Check sheet for the modelled part. Datum: model origin and axes. Units: mm. A direction names the side the tool comes from. Round coordinates to 2 decimals unless told otherwise and drop trailing zeros. Order: outer loops, then holes, each group sorted by start corner. A loop starts at its lowest first (then second) coordinate and runs counter-clockwise, first axis right, second up. Notation, with made-up numbers: (-27, 10.25) -> (-3, 10.25) arc R34 ccw to (-3, 44.25) -> close; hole circle Ø10 at (40, 73.25). An arc over 180 degrees is marked (long way). Answer in a Markdown table with one row per item. Add a question column.
1. Access from +Z, -Z, +X, -X, +Y, -Y to the whole of each face (thin tool, end or side, straight path). Record for faces 4 (the flat face through (7, 5, -7.5)), 5 (the cylindrical face through (31.21, 2.96, -17.94)).
2. Draft check along X on faces 1 (the cylindrical face through (-21.28, 2.96, 21.15)), 2 (the flat face through (-19, 6, 0)), 3 (the cylindrical face through (-31.21, 2.96, 17.94)). Enter one of: +X half, -X half, draft (parallel to the pull), parting line (faces both ways), or undercut.
3. Material ranges on L1, parallel to X at y = 1.05, z = -30; L2, parallel to Z at x = 16, y = 4.3; L3, parallel to Z at x = 30.5, y = 2.4, recorded low to high. Write a range as from..to.
4. Sectioned sample at A-A, the plane y = 2.3. Record the boundary of the cut face in (x, z).
5. Depth check by flat-ended pin: P1, Ø2, axis at y = 4.5, z = 10, coming from the -X side; P2, Ø1.9, axis at y = 5, z = 4, coming from the +X side; P3, Ø1, axis at y = 4.5, z = -2.5, coming from the -X side. Enter the tip coordinate at first touch or a pass-through.
6. Sectioned sample at B-B, the plane x = 7. Record the boundary of the cut face in (y, z), then the cut area to 3 significant figures.
```python
from build123d import *

# Parameters (mm, degrees)
BOSS_EXTRUDE1_DEPTH = 4
BOSS_EXTRUDE3_DEPTH = 2
CUT_EXTRUDE1_DEPTH  = 2
SKETCH2_R           = 26
SKETCH2_R_2         = 24
BOSS_EXTRUDE4_DEPTH = 2
SKETCH5_W           = 30
SKETCH5_H           = 15
SKETCH5_R           = 4
SKETCH5_R_2         = 2
BOSS_EXTRUDE5_DEPTH = 2
BOSS_EXTRUDE6_DEPTH = 2
CUT_EXTRUDE2_DEPTH  = 2
SKETCH8_R           = 2
CUT_EXTRUDE3_DEPTH  = 6
FILLET1_R           = 2


with BuildPart() as part:
    # Sketch1 → Boss-Extrude1 (new body)
    with BuildSketch(Plane(origin=(0, 0, 0), x_dir=(1, 0, 0), z_dir=(0, 1, 0))):
        with BuildLine():
            ThreePointArc((31.766819559, 13.412064474), (28.977774789, 7.764571353), (34.216904973, 4.268221228))
            ThreePointArc((34.216904973, 4.268221228), (36, 0), (34.216904973, -4.268221228))
            ThreePointArc((34.216904973, -4.268221228), (28.977774789, -7.764571353), (31.766819559, -13.412064474))
            ThreePointArc((31.766819559, -13.412064474), (31.176914536, -18), (27.498598332, -20.804840499))
            ThreePointArc((27.498598332, -20.804840499), (21.213203436, -21.213203436), (20.804840499, -27.498598332))
            ThreePointArc((20.804840499, -27.498598332), (18, -31.176914536), (13.412064474, -31.766819559))
            ThreePointArc((13.412064474, -31.766819559), (7.764571353, -28.977774789), (4.268221228, -34.216904973))
            ThreePointArc((4.268221228, -34.216904973), (0, -36), (-4.268221228, -34.216904973))
            ThreePointArc((-4.268221228, -34.216904973), (-7.764571353, -28.977774789), (-13.412064474, -31.766819559))
            ThreePointArc((-13.412064474, -31.766819559), (-18, -31.176914536), (-20.804840499, -27.498598332))
            ThreePointArc((-20.804840499, -27.498598332), (-21.213203436, -21.213203436), (-27.498598332, -20.804840499))
            ThreePointArc((-27.498598332, -20.804840499), (-31.176914536, -18), (-31.766819559, -13.412064474))
            ThreePointArc((-31.766819559, -13.412064474), (-28.977774789, -7.764571353), (-34.216904973, -4.268221228))
            ThreePointArc((-34.216904973, -4.268221228), (-36, 0), (-34.216904973, 4.268221228))
            ThreePointArc((-34.216904973, 4.268221228), (-28.977774789, 7.764571353), (-31.766819559, 13.412064474))
            ThreePointArc((-31.766819559, 13.412064474), (-31.176914536, 18), (-27.498598332, 20.804840499))
            ThreePointArc((-27.498598332, 20.804840499), (-21.213203436, 21.213203436), (-20.804840499, 27.498598332))
            ThreePointArc((-20.804840499, 27.498598332), (-18, 31.176914536), (-13.412064474, 31.766819559))
            ThreePointArc((-13.412064474, 31.766819559), (-7.764571353, 28.977774789), (-4.268221228, 34.216904973))
            ThreePointArc((-4.268221228, 34.216904973), (0, 36), (4.268221228, 34.216904973))
            ThreePointArc((4.268221228, 34.216904973), (7.764571353, 28.977774789), (13.412064474, 31.766819559))
            ThreePointArc((13.412064474, 31.766819559), (18, 31.176914536), (20.804840499, 27.498598332))
            ThreePointArc((20.804840499, 27.498598332), (21.213203436, 21.213203436), (27.498598332, 20.804840499))
            ThreePointArc((27.498598332, 20.804840499), (31.176914536, 18), (31.766819559, 13.412064474))
        make_face()
    extrude(amount=BOSS_EXTRUDE1_DEPTH)

    # Sketch4 → Boss-Extrude3 (add)
    with BuildSketch(Plane(origin=(0, 4, 0), x_dir=(1, 0, 0), z_dir=(0, 1, 0))):
        with BuildLine():
            ThreePointArc((-13.412064474, 31.766819559), (-18, 31.176914536), (-20.804840499, 27.498598332))
            ThreePointArc((-20.804840499, 27.498598332), (-21.213203436, 21.213203436), (-27.498598332, 20.804840499))
            ThreePointArc((-27.498598332, 20.804840499), (-31.176914536, 18), (-31.766819559, 13.412064474))
            ThreePointArc((-31.766819559, 13.412064474), (-28.977774789, 7.764571353), (-34.216904973, 4.268221228))
            ThreePointArc((-34.216904973, 4.268221228), (-36, 0), (-34.216904973, -4.268221228))
            ThreePointArc((-34.216904973, -4.268221228), (-28.977774789, -7.764571353), (-31.766819559, -13.412064474))
            ThreePointArc((-31.766819559, -13.412064474), (-31.176914536, -18), (-27.498598332, -20.804840499))
            ThreePointArc((-27.498598332, -20.804840499), (-21.213203436, -21.213203436), (-20.804840499, -27.498598332))
            ThreePointArc((-20.804840499, -27.498598332), (-18, -31.176914536), (-13.412064474, -31.766819559))
            ThreePointArc((-13.412064474, -31.766819559), (-7.764571353, -28.977774789), (-4.268221228, -34.216904973))
            ThreePointArc((-4.268221228, -34.216904973), (0, -36), (4.268221228, -34.216904973))
            ThreePointArc((4.268221228, -34.216904973), (7.764571353, -28.977774789), (13.412064474, -31.766819559))
            ThreePointArc((13.412064474, -31.766819559), (18, -31.176914536), (20.804840499, -27.498598332))
            ThreePointArc((20.804840499, -27.498598332), (21.213203436, -21.213203436), (27.498598332, -20.804840499))
            ThreePointArc((27.498598332, -20.804840499), (31.176914536, -18), (31.766819559, -13.412064474))
            ThreePointArc((31.766819559, -13.412064474), (28.977774789, -7.764571353), (34.216904973, -4.268221228))
            ThreePointArc((34.216904973, -4.268221228), (36, 0), (34.216904973, 4.268221228))
            ThreePointArc((34.216904973, 4.268221228), (28.977774789, 7.764571353), (31.766819559, 13.412064474))
            ThreePointArc((31.766819559, 13.412064474), (31.176914536, 18), (27.498598332, 20.804840499))
            ThreePointArc((27.498598332, 20.804840499), (21.213203436, 21.213203436), (20.804840499, 27.498598332))
            ThreePointArc((20.804840499, 27.498598332), (18, 31.176914536), (13.412064474, 31.766819559))
            ThreePointArc((13.412064474, 31.766819559), (7.764571353, 28.977774789), (4.268221228, 34.216904973))
            ThreePointArc((4.268221228, 34.216904973), (0, 36), (-4.268221228, 34.216904973))
            ThreePointArc((-4.268221228, 34.216904973), (-7.764571353, 28.977774789), (-13.412064474, 31.766819559))
        make_face()
    extrude(amount=BOSS_EXTRUDE3_DEPTH)

    # Sketch3 → Cut-Extrude1 (cut)
    with BuildSketch(Plane(origin=(0, 4, 0), x_dir=(1, 0, 0), z_dir=(0, 1, 0))):
        with BuildLine():
            ThreePointArc((-14.726691345, 29.971413987), (-17, 29.444863729), (-18.592660228, 27.739395812))
            ThreePointArc((-18.592660228, 27.739395812), (-19.798989873, 19.798989873), (-27.739395812, 18.592660228))
            ThreePointArc((-27.739395812, 18.592660228), (-29.444863729, 17), (-29.971413987, 14.726691345))
            ThreePointArc((-29.971413987, 14.726691345), (-27.045923136, 7.246933263), (-33.319351573, 2.232018175))
            ThreePointArc((-33.319351573, 2.232018175), (-34, 0), (-33.319351573, -2.232018175))
            ThreePointArc((-33.319351573, -2.232018175), (-27.045923136, -7.246933263), (-29.971413987, -14.726691345))
            ThreePointArc((-29.971413987, -14.726691345), (-29.444863729, -17), (-27.739395812, -18.592660228))
            ThreePointArc((-27.739395812, -18.592660228), (-19.798989873, -19.798989873), (-18.592660228, -27.739395812))
            ThreePointArc((-18.592660228, -27.739395812), (-17, -29.444863729), (-14.726691345, -29.971413987))
            ThreePointArc((-14.726691345, -29.971413987), (-7.246933263, -27.045923136), (-2.232018175, -33.319351573))
            ThreePointArc((-2.232018175, -33.319351573), (0, -34), (2.232018175, -33.319351573))
            ThreePointArc((2.232018175, -33.319351573), (7.246933263, -27.045923136), (14.726691345, -29.971413987))
            ThreePointArc((14.726691345, -29.971413987), (17, -29.444863729), (18.592660228, -27.739395812))
            ThreePointArc((18.592660228, -27.739395812), (19.798989873, -19.798989873), (27.739395812, -18.592660228))
            ThreePointArc((27.739395812, -18.592660228), (29.444863729, -17), (29.971413987, -14.726691345))
            ThreePointArc((29.971413987, -14.726691345), (27.045923136, -7.246933263), (33.319351573, -2.232018175))
            ThreePointArc((33.319351573, -2.232018175), (34, 0), (33.319351573, 2.232018175))
            ThreePointArc((33.319351573, 2.232018175), (27.045923136, 7.246933263), (29.971413987, 14.726691345))
            ThreePointArc((29.971413987, 14.726691345), (29.444863729, 17), (27.739395812, 18.592660228))
            ThreePointArc((27.739395812, 18.592660228), (19.798989873, 19.798989873), (18.592660228, 27.739395812))
            ThreePointArc((18.592660228, 27.739395812), (17, 29.444863729), (14.726691345, 29.971413987))
            ThreePointArc((14.726691345, 29.971413987), (7.246933263, 27.045923136), (2.232018175, 33.319351573))
            ThreePointArc((2.232018175, 33.319351573), (0, 34), (-2.232018175, 33.319351573))
            ThreePointArc((-2.232018175, 33.319351573), (-7.246933263, 27.045923136), (-14.726691345, 29.971413987))
        make_face()
    extrude(amount=CUT_EXTRUDE1_DEPTH, mode=Mode.SUBTRACT)

    # Sketch2 → Boss-Extrude4 (add)
    with BuildSketch(Plane(origin=(0, 4, 0), x_dir=(1, 0, 0), z_dir=(0, 1, 0))):
        with Locations(Location((0, 0, 0), (0, 0, 270))):
            Circle(SKETCH2_R)
        with Locations(Location((0, 0, 0), (0, 0, 270))):
            Circle(SKETCH2_R_2, mode=Mode.SUBTRACT)
    extrude(amount=BOSS_EXTRUDE4_DEPTH)

    # Sketch5 → Boss-Extrude5 (add)
    # profile 1 of 5: a face of its own
    with BuildSketch(Plane(origin=(0, 4, 0), x_dir=(1, 0, 0), z_dir=(0, 1, 0))):
        with BuildLine():
            Line((-17, 5), (-17, -5))
            ThreePointArc((-17, -5), (-22, 0), (-17, 5))
        make_face()
    # profile 2 of 5: a face of its own
    with BuildSketch(Plane(origin=(0, 4, 0), x_dir=(1, 0, 0), z_dir=(0, 1, 0))):
        Rectangle(SKETCH5_W, SKETCH5_H)
        with Locations(Location((-7, 0, 0), (0, 0, 270))):
            Circle(SKETCH5_R, mode=Mode.SUBTRACT)
        with Locations(Location((7, 0, 0), (0, 0, 270))):
            Circle(SKETCH5_R, mode=Mode.SUBTRACT)
    # profile 3 of 5: a face of its own
    with BuildSketch(Plane(origin=(0, 4, 0), x_dir=(1, 0, 0), z_dir=(0, 1, 0))):
        with Locations(Location((-7, 0, 0), (0, 0, 270))):
            Circle(SKETCH5_R_2)
    # profile 4 of 5: a face of its own
    with BuildSketch(Plane(origin=(0, 4, 0), x_dir=(1, 0, 0), z_dir=(0, 1, 0))):
        with Locations(Location((7, 0, 0), (0, 0, 270))):
            Circle(SKETCH5_R_2)
    # profile 5 of 5: a face of its own
    with BuildSketch(Plane(origin=(0, 4, 0), x_dir=(1, 0, 0), z_dir=(0, 1, 0))):
        with BuildLine():
            ThreePointArc((17, 5), (22, 0), (17, -5))
            Line((17, -5), (17, 5))
        make_face()
    extrude(amount=BOSS_EXTRUDE5_DEPTH)

    # Sketch6 → Boss-Extrude6 (add)
    with BuildSketch(Plane(origin=(0, 4, 0), x_dir=(1, 0, 0), z_dir=(0, 1, 0))):
        with BuildLine():
            Line((0, 7.5), (1.907283427, 12.740218147))
            ThreePointArc((1.907283427, 12.740218147), (4.07818129, 15.957233587), (3.67332787, 12.097430538))
            Line((3.67332787, 12.097430538), (2, 7.5))
            Line((2, 7.5), (0, 7.5))
        make_face()
    extrude(amount=BOSS_EXTRUDE6_DEPTH)

    # Sketch7 → Cut-Extrude2 (cut)
    with BuildSketch(Plane(origin=(0, 6, 0), x_dir=(1, 0, 0), z_dir=(0, 1, 0))):
        with BuildLine():
            Line((2.126154469, -3.388136239), (2.510116854, -4))
            Line((2.510116854, -4), (2.973799982, -4.738902857))
            ThreePointArc((2.973799982, -4.738902857), (0.649911516, -5.55682478), (-1.8, -5.297233865))
            Line((-1.8, -5.297233865), (-1.8, -3.57211422))
            ThreePointArc((-1.8, -3.57211422), (0.1872329, -3.995615577), (2.126154469, -3.388136239))
        make_face()
    extrude(amount=-CUT_EXTRUDE2_DEPTH, mode=Mode.SUBTRACT)

    # Sketch8 → Cut-Extrude3 (cut)
    with BuildSketch(Plane(origin=(0, 4, 0), x_dir=(1, 0, 0), z_dir=(0, 1, 0))):
        with Locations(Location((0, 30, 0), (0, 0, 270))):
            Circle(SKETCH8_R)
    extrude(amount=-CUT_EXTRUDE3_DEPTH, mode=Mode.SUBTRACT)

    # Fillet1
    fillet1_edges = [part.edges().sort_by_distance(p)[0] for p in [
        (-15, 5, 7.5),
        (15, 5, 7.5),
        (15, 5, -7.5),
        (-15, 5, -7.5),
    ]]
    fillet(fillet1_edges, radius=FILLET1_R)


solid = part.part
```
Answer key:
| question | item | result |
|---|---|---|
| 1 | face 4 | +Y |
| 1 | face 5 | +X, +Y, -Y |
| 2 | face 1 | undercut |
| 2 | face 2 | draft |
| 2 | face 3 | -X half |
| 3 | L1 | x = -19.45..-12.15, -5.85..-2, 2..5.85, 12.15..19.45 |
| 3 | L2 | z = -31.9..-29.85, -20.49..-17.89, 17.89..20.49, 29.85..31.9 |
| 3 | L3 | z = -18.95..-12.64, -5.36..5.36, 12.64..18.95 |
| 4 | outline | (-34.22, -4.27) arc R4.77 cw to (-31.77, -13.41) arc R6 ccw to (-27.5, -20.8) arc R4.77 cw to (-20.8, -27.5) arc R6 ccw to (-13.41, -31.77) arc R4.77 cw to (-4.27, -34.22) arc R6 ccw to (4.27, -34.22) arc R4.77 cw to (13.41, -31.77) arc R6 ccw to (20.8, -27.5) arc R4.77 cw to (27.5, -20.8) arc R6 ccw to (31.77, -13.41) arc R4.77 cw to (34.22, -4.27) arc R6 ccw to (34.22, 4.27) arc R4.77 cw to (31.77, 13.41) arc R6 ccw to (27.5, 20.8) arc R4.77 cw to (20.8, 27.5) arc R6 ccw to (13.41, 31.77) arc R4.77 cw to (4.27, 34.22) arc R6 ccw to (-4.27, 34.22) arc R4.77 cw to (-13.41, 31.77) arc R6 ccw to (-20.8, 27.5) arc R4.77 cw to (-27.5, 20.8) arc R6 ccw to (-31.77, 13.41) arc R4.77 cw to (-34.22, 4.27) arc R6 ccw to start; hole circle Ø4 at (0, -30) |
| 5 | P1 | stops at x = -29.25 |
| 5 | P2 | stops at x = 35.17 |
| 5 | P3 | stops at x = -35.66 |
| 6 | outline | (0, -29.25) -> (6, -29.25) -> (6, -27.12) -> (4, -27.12) -> (4, -25.04) -> (6, -25.04) -> (6, -22.96) -> (4, -22.96) -> (4, -7.5) -> (6, -7.5) -> (6, -4) -> (4, -4) -> (4, -2) -> (6, -2) -> (6, 2) -> (4, 2) -> (4, 4) -> (6, 4) -> (6, 7.5) -> (4, 7.5) -> (4, 22.96) -> (6, 22.96) -> (6, 25.04) -> (4, 25.04) -> (4, 27.12) -> (6, 27.12) -> (6, 29.25) -> (0, 29.25) -> close |
| 6 | area | 273 mm² |
